Could you check a few things on this model? Use its own coordinates, in mm. Give positions to 0.01 mm unless a question says otherwise; leave off trailing zeros. Write each loop counter-clockwise with the first axis right and the second up, starting at its lowest first coordinate (ties: lowest second). Pieces come first, ordered by that corner, then holes. Notation, with made-up numbers: (-23, -2.5) - (11, -2.5) arc R25 cw to (11, 19.5) - close; hole circle Ø3 at (76.25, 44). An arc over 180 degrees is marked (long way). Use one line per item in the form item = value.
```python
from build123d import *

# Parameters (mm, degrees)
F0_W     = 50
F0_H     = 25
F1_DEPTH = 8
F2_R     = 5.25
F3_DEPTH = 8.001


with BuildPart() as f1:
    # F0 (on Top) → F1 (new body)
    with BuildSketch(Plane.XY):
        Rectangle(F0_W, F0_H)
    extrude(amount=-F1_DEPTH)

    # F2 (on face) → F3 (cut, through all)
    with BuildSketch(Plane.XY):
        Circle(F2_R)
    extrude(amount=-F3_DEPTH, mode=Mode.SUBTRACT)


solid = f1.part
```
1. Imagine slicing it at A-A, the plane y = 0. List the corners of the cut face in (x, z) for me, and give its area (3 significant figures).
Response values:
outline = (-25, -8) - (-5.25, -8) - (-5.25, 0) - (-25, 0) - close; (5.25, -8) - (25, -8) - (25, 0) - (5.25, 0) - close
area = 316 mm²
2. If I drill on line 1 (Y direction, x = 0, z = -3); line 2 (X direction, y = -1, z = -5.25); line 3 (X direction, y = 3.5, z = -0.25), over which ranges is the centre line in solid material (lowest first)? Write a range as from..to.
Response values:
line_1 = -12.5..-5.25, 5.25..12.5
line_2 = -25..-5.15, 5.15..25
line_3 = -25..-3.91, 3.91..25
3. Imagine slicing it at C-C, the plane z = -2.5. List the corners of the cut face in (x, y) for me.
Response values:
outline = (-25, -12.5) - (25, -12.5) - (25, 12.5) - (-25, 12.5) - close; hole circle Ø10.5 at (0, 0)
4. If we mould it in two halves opening along X, with no side actions, what happens to faces 1 (the face through (25, 0, -4)), 2 (the face through (0, 12.5, -4)), 3 (the face through (5, 1.6, -3.9))? For each: pulls with the +X half, pulls with the -X half, needs draft (parallel to the pull), parting line crosses it, or undercut.
Response values:
face_1 = pulls with the +X half
face_2 = needs draft
face_3 = undercut
5. Imagine slicing it at B-B, the plane x = 0. List the corners of the cut face in (y, z) for me, and give its area (3 significant figures).
Response values:
outline = (-12.5, -8) - (-5.25, -8) - (-5.25, 0) - (-12.5, 0) - close; (5.25, -8) - (12.5, -8) - (12.5, 0) - (5.25, 0) - close
area = 116 mm²
6. For pin 1 (12 mm diameter, centred on x = 0, y = 0, fed in from -Z), with a flat end and sliding along its axis, tell me the tip position at first contact or that it passes through.
Response values:
pin_1 = -8
